```python
from build123d import *

# Parameters (mm, degrees)
SKETCH1_W                 = 52.5
SKETCH1_H                 = 2
SKETCH2_W                 = 4
SKETCH2_H                 = 7
SKETCH3_W                 = 4
SKETCH3_H                 = 7
SKETCH4_W                 = 4
SKETCH4_H                 = 7
SKETCH5_W                 = 4
SKETCH5_H                 = 7
SKETCH6_W                 = 4
SKETCH6_H                 = 7
SKETCH7_W                 = 4
SKETCH7_H                 = 7
F_4_0_4_DIAMETER_HOLE1_D  = 4
M80_CLEARANCE_HOLE1_D     = 85
M80_CLEARANCE_HOLE1_DEPTH = 9
CHAMFER1_SIZE             = 0.5


with BuildPart() as part:
    # Sketch1 → Revolve1 (revolve)
    with BuildSketch(Plane.XZ, mode=Mode.PRIVATE) as revolve1_sk:
        with Locations((26.25, 1)):
            Rectangle(SKETCH1_W, SKETCH1_H)
    revolve(revolve1_sk.sketch.rotate(Axis((0, 0, 2), (0, 0, -1)), 180), axis=Axis((0, 0, 2), (0, 0, -1)))

    # Sketch2 → Revolve2 (revolve)
    with BuildSketch(Plane.XZ.offset(23.75), mode=Mode.PRIVATE) as revolve2_sk:
        with Locations((43.13620668, 5.5)):
            Rectangle(SKETCH2_W, SKETCH2_H)
    revolve(revolve2_sk.sketch.rotate(Axis((41.13620668, -23.75, 9), (0, 0, -1)), 180), axis=Axis((41.13620668, -23.75, 9), (0, 0, -1)))

    # Sketch3 → Revolve3 (revolve)
    with BuildSketch(Plane.XZ.offset(23.75), mode=Mode.PRIVATE) as revolve3_sk:
        with Locations((-39.13620668, 5.5)):
            Rectangle(SKETCH3_W, SKETCH3_H)
    revolve(revolve3_sk.sketch.rotate(Axis((-41.13620668, -23.75, 9), (0, 0, -1)), 180), axis=Axis((-41.13620668, -23.75, 9), (0, 0, -1)))

    # Sketch4 → Revolve4 (revolve)
    with BuildSketch(Plane.XZ.offset(-47.5), mode=Mode.PRIVATE) as revolve4_sk:
        with Locations((2, 5.5)):
            Rectangle(SKETCH4_W, SKETCH4_H)
    revolve(revolve4_sk.sketch.rotate(Axis((0, 47.5, 9), (0, 0, -1)), 180), axis=Axis((0, 47.5, 9), (0, 0, -1)))

    # Sketch5 → Revolve5 (revolve)
    with BuildSketch(Plane(origin=(0, 23.75, 0), x_dir=(1, 0, 0), z_dir=(0, 1, 0))):
        with Locations((43.13620668, 3.5)):
            Rectangle(SKETCH5_W, SKETCH5_H)
    revolve(axis=Axis((41.13620668, 23.75, -7), (0, 0, 1)))

    # Sketch6 → Revolve6 (revolve)
    with BuildSketch(Plane(origin=(0, 23.75, 0), x_dir=(1, 0, 0), z_dir=(0, 1, 0))):
        with Locations((-39.13620668, 3.5)):
            Rectangle(SKETCH6_W, SKETCH6_H)
    revolve(axis=Axis((-41.13620668, 23.75, -7), (0, 0, 1)))

    # Sketch7 → Revolve7 (revolve)
    with BuildSketch(Plane(origin=(0, -47.5, 0), x_dir=(1, 0, 0), z_dir=(0, 1, 0))):
        with Locations((2, 3.5)):
            Rectangle(SKETCH7_W, SKETCH7_H)
    revolve(axis=Axis((0, -47.5, -7), (0, 0, 1)))

    # Sketch8 → Cut-Revolve1 (revolve, cut)
    with BuildSketch(Plane(origin=(0, 47.5, 0), x_dir=(1, 0, 0), z_dir=(0, 1, 0))):
        Polygon((1.2295, 0), (0, 0), (0, -9), (1.2295, -9), (1.2295, -7), align=None)
    revolve(axis=Axis((0, 47.5, 0), (0, 0, 1)), mode=Mode.SUBTRACT)

    # Sketch9 → Cut-Revolve2 (revolve, cut)
    with BuildSketch(Plane(origin=(0, -23.75, 0), x_dir=(1, 0, 0), z_dir=(0, 1, 0))):
        Polygon((-39.90670668, 0), (-41.13620668, 0), (-41.13620668, -9), (-39.90670668, -9), (-39.90670668, -7), align=None)
    revolve(axis=Axis((-41.13620668, -23.75, 0), (0, 0, 1)), mode=Mode.SUBTRACT)

    # Sketch10 → Cut-Revolve3 (revolve, cut)
    with BuildSketch(Plane(origin=(0, -23.75, 0), x_dir=(1, 0, 0), z_dir=(0, 1, 0))):
        Polygon((42.36570668, 0), (41.13620668, 0), (41.13620668, -9), (42.36570668, -9), (42.36570668, -7), align=None)
    revolve(axis=Axis((41.13620668, -23.75, 0), (0, 0, 1)), mode=Mode.SUBTRACT)

    # Ø4.0 (4) Diameter Hole1 (through all)
    with Locations(Plane(origin=(0, 0, -7), x_dir=(-1, 0, 0), z_dir=(0, 0, -1))):
        with Locations((-41.13620668, 23.75), (0, -47.5), (41.13620668, 23.75)):
            Hole(F_4_0_4_DIAMETER_HOLE1_D / 2)

    # M80 Clearance Hole1
    with Locations(Plane.XY.offset(2)):
        with Locations((0, 0)):
            Hole(M80_CLEARANCE_HOLE1_D / 2, depth=M80_CLEARANCE_HOLE1_DEPTH)

    # Chamfer1
    chamfer1_edges = [part.edges().sort_by_distance(p)[0] for p in [
        (52.5, 0, 0),
        (52.5, 0, 2),
        (42.5, 0, 0),
        (42.5, 0, 2),
    ]]
    chamfer(chamfer1_edges, length=CHAMFER1_SIZE)


solid = part.part
```
Can you work these out from the model? Positions are in its coordinate system, mm. A direction names the side the tool comes from. Round coordinates to 2 decimals unless told otherwise and drop trailing zeros. Loops run counter-clockwise (first coordinate to the right, second up) from the corner with the lowest first, then second, coordinate; pieces in that order, holes last. Notation, with made-up numbers: (82.25, 4.5) -> (127.25, 4.5) arc R11 ccw to (127.25, 14.5) -> close; hole circle Ø6 at (38, -12). An arc over 180 degrees is marked (long way). One line per item, written item: value. Start each with the question number.
1. For pin 1 (3 mm diameter, centred on x = -41.14, y = -23.75, fed in from -Z); pin 2 (5 mm diameter, centred on x = -25.5, z = 1.5, fed in from -Y); pin 3 (6 mm diameter, centred on x = 3.5, z = 6.5, fed in from +Y), each with a flat end and sliding along its axis, tell me the tip position at first contact or that it passes through.
2. If we mould it in two halves opening along Y, with no side actions, what happens to faces 1 (the cylindrical face through (-37.32, 24.95, -3.55)), 2 (the flat face through (-20, 39, 2)), 3 (the cylindrical face through (-0.16, 48.72, 4.44))? For each: pulls with the +Y half, pulls with the -Y half, needs draft (parallel to the pull), parting line crosses it, or undercut.
3. If I drill on probe 1 along Y at (x, z) = (0, 1.05); probe 2 along Y at (x, z) = (0, -2.5); probe 3 along Z at (x, y) = (-33.5, -39.5), over which ranges is the centre line in solid material (lowest first)?
4. For faces 4 (the cylindrical face through (39.908, -23.696, 4.437)), 5 (the cylindrical face through (37.32, -22.55, 5.55)), 6 (the cylindrical face through (44.95, 24.95, -3.55)), which set-ups out of +Z, -Z, +X, -X, +Y, -Y let a thin tool reach every point of the face, with its end or its side?
5. If we section it at B-B, the plane y = 0: Write out the boundary of the cut face in (x, z).
6. If we section it at C-C, the plane x = 0: Give the number of separate pieces and of enclosed holes in the cut face, then the cut area to 3 significant figures.
7. If we section it at A-A, the plane z = 6.5: Write out the boundary of the cut face in (x, y), then the cut area to 3 significant figures.
Calculated:
1. pin 1: stops at z = 0
1. pin 2: stops at y = -47.19
1. pin 3: stops at y = 51.47
2. face 1: parting line crosses it
2. face 2: needs draft
2. face 3: undercut
3. probe 1: y = -52.5 to -49.5, -45.5 to -42.5, 42.5 to 46.27, 48.73 to 52.5
3. probe 2: y = -51.5 to -49.5, -45.5 to -43.5
3. probe 3: z = 0 to 2
4. face 4: +Z, -Z
4. face 5: +Z
4. face 6: -Z
5. outline: (-52.5, 0.5) -> (-52, 0) -> (-43, 0) -> (-42.5, 0.5) -> (-42.5, 1.5) -> (-43, 2) -> (-52, 2) -> (-52.5, 1.5) -> close; (42.5, 0.5) -> (43, 0) -> (52, 0) -> (52.5, 0.5) -> (52.5, 1.5) -> (52, 2) -> (43, 2) -> (42.5, 1.5) -> close
6. separate pieces: 4
6. enclosed holes: 0
6. area: 92.9 mm²
7. outline: circle Ø8 at (-41.14, -23.75); circle Ø8 at (0, 47.5); circle Ø8 at (41.14, -23.75); hole circle Ø2.46 at (-41.14, -23.75); hole circle Ø2.46 at (0, 47.5); hole circle Ø2.46 at (41.14, -23.75)
7. area: 137 mm²
